```python
from build123d import *

# Parameters (mm, degrees)
SKETCH1_W                                    = 80
SKETCH1_H                                    = 225
BOSS_EXTRUDE1_DEPTH                          = 20
CUT_EXTRUDE1_REACH                           = 123.063
CUT_EXTRUDE2_DEPTH                           = 5
CBORE_FOR_M8_HEX_SOCKET_HEAD_CAP_SCR_2_COUNT = 2
CBORE_FOR_M8_HEX_SOCKET_HEAD_CAP_SCR_2_PITCH = 50
CBORE_FOR_M8_HEX_SOCKET_HEAD_CAP_SCR_3_COUNT = 2
CBORE_FOR_M8_HEX_SOCKET_HEAD_CAP_SCR_3_PITCH = 201.308221392
CBORE_FOR_M8_HEX_SOCKET_HEAD_CAP_SCR_4_COUNT = 2
CBORE_FOR_M8_HEX_SOCKET_HEAD_CAP_SCR_4_PITCH = 195
F_8_0MM_DOWEL_HOLE1_D                        = 8
SKETCH11_R                                   = 10
CUT_EXTRUDE3_DEPTH                           = 122.063000128
CUT_EXTRUDE4_REACH                           = 123.063
SKETCH13_R                                   = 6
CUT_EXTRUDE5_REACH                           = 123.063
SKETCH14_R                                   = 7


with BuildPart() as part:
    # Sketch1 → Boss-Extrude1 (new body)
    with BuildSketch(Plane(origin=(0, 0, 0), x_dir=(1, 0, 0), z_dir=(0, 1, 0))):
        Rectangle(SKETCH1_W, SKETCH1_H)
    extrude(amount=-BOSS_EXTRUDE1_DEPTH)

    # Sketch2 → Cut-Extrude1 (cut, up to next)
    with BuildSketch(Plane(origin=(0, 0, 0), x_dir=(1, 0, 0), z_dir=(0, 1, 0)), mode=Mode.PRIVATE) as cut_extrude1_sk1:
        with BuildLine():
            Line((24, 17.31), (24, 34.91))
            ThreePointArc((24, 34.91), (21.5, 37.41), (19, 34.91))
            Line((19, 34.91), (19, 17.31))
            ThreePointArc((19, 17.31), (21.5, 14.81), (24, 17.31))
        make_face()
    cut_extrude1_tool1 = extrude(cut_extrude1_sk1.sketch, amount=-CUT_EXTRUDE1_REACH, mode=Mode.PRIVATE) & part.part
    # Sketch2 → Cut-Extrude1 (cut, up to next)
    with BuildSketch(Plane(origin=(0, 0, 0), x_dir=(1, 0, 0), z_dir=(0, 1, 0)), mode=Mode.PRIVATE) as cut_extrude1_sk2:
        with BuildLine():
            Line((24, -36.69), (24, -12.59))
            ThreePointArc((24, -12.59), (21.5, -10.09), (19, -12.59))
            Line((19, -12.59), (19, -36.69))
            ThreePointArc((19, -36.69), (21.5, -39.19), (24, -36.69))
        make_face()
    cut_extrude1_tool2 = extrude(cut_extrude1_sk2.sketch, amount=-CUT_EXTRUDE1_REACH, mode=Mode.PRIVATE) & part.part
    # Sketch2 → Cut-Extrude1 (cut, up to next)
    with BuildSketch(Plane(origin=(0, 0, 0), x_dir=(1, 0, 0), z_dir=(0, 1, 0)), mode=Mode.PRIVATE) as cut_extrude1_sk3:
        with BuildLine():
            Line((-24, -16.59), (-24, -36.69))
            ThreePointArc((-24, -36.69), (-21.5, -39.19), (-19, -36.69))
            Line((-19, -36.69), (-19, -16.59))
            ThreePointArc((-19, -16.59), (-21.5, -14.09), (-24, -16.59))
        make_face()
    cut_extrude1_tool3 = extrude(cut_extrude1_sk3.sketch, amount=-CUT_EXTRUDE1_REACH, mode=Mode.PRIVATE) & part.part
    # Sketch2 → Cut-Extrude1 (cut, up to next)
    with BuildSketch(Plane(origin=(0, 0, 0), x_dir=(1, 0, 0), z_dir=(0, 1, 0)), mode=Mode.PRIVATE) as cut_extrude1_sk4:
        with BuildLine():
            Line((-24, 53.91), (-24, 36.31))
            ThreePointArc((-24, 36.31), (-21.5, 33.81), (-19, 36.31))
            Line((-19, 36.31), (-19, 53.91))
            ThreePointArc((-19, 53.91), (-21.5, 56.41), (-24, 53.91))
        make_face()
    cut_extrude1_tool4 = extrude(cut_extrude1_sk4.sketch, amount=-CUT_EXTRUDE1_REACH, mode=Mode.PRIVATE) & part.part
    add(cut_extrude1_tool1.solids().sort_by_distance((21.5, 0, -26.11))[0], mode=Mode.SUBTRACT)
    add(cut_extrude1_tool2.solids().sort_by_distance((21.5, 0, 24.64))[0], mode=Mode.SUBTRACT)
    add(cut_extrude1_tool3.solids().sort_by_distance((-21.5, 0, 26.64))[0], mode=Mode.SUBTRACT)
    add(cut_extrude1_tool4.solids().sort_by_distance((-21.5, 0, -45.11))[0], mode=Mode.SUBTRACT)

    # Sketch3 → Cut-Extrude2 (cut)
    with BuildSketch(Plane(origin=(0, 0, 0), x_dir=(1, 0, 0), z_dir=(0, 1, 0))):
        with BuildLine():
            Line((-17.5, 36.31), (-17.5, 53.91))
            ThreePointArc((-17.5, 53.91), (-21.5, 57.91), (-25.5, 53.91))
            Line((-25.5, 53.91), (-25.5, 36.31))
            ThreePointArc((-25.5, 36.31), (-21.5, 32.31), (-17.5, 36.31))
        make_face()
        with BuildLine():
            Line((25.5, 17.31), (25.5, 34.91))
            ThreePointArc((25.5, 34.91), (21.5, 38.91), (17.5, 34.91))
            Line((17.5, 34.91), (17.5, 17.31))
            ThreePointArc((17.5, 17.31), (21.5, 13.31), (25.5, 17.31))
        make_face()
        with BuildLine():
            Line((25.5, -36.69), (25.5, -12.59))
            ThreePointArc((25.5, -12.59), (21.5, -8.59), (17.5, -12.59))
            Line((17.5, -12.59), (17.5, -36.69))
            ThreePointArc((17.5, -36.69), (21.5, -40.69), (25.5, -36.69))
        make_face()
        with BuildLine():
            Line((-25.5, -16.59), (-25.5, -36.69))
            ThreePointArc((-25.5, -36.69), (-21.5, -40.69), (-17.5, -36.69))
            Line((-17.5, -36.69), (-17.5, -16.59))
            ThreePointArc((-17.5, -16.59), (-21.5, -12.59), (-25.5, -16.59))
        make_face()
    extrude(amount=-CUT_EXTRUDE2_DEPTH, mode=Mode.SUBTRACT)

    # Sketch6 → CBORE for M8 Hex Socket Head Cap Screw1 (revolve, cut)
    with BuildSketch(Plane(origin=(25, -20, -97.5), x_dir=(0, 0, -1), z_dir=(1, 0, 0))):
        Polygon((0, 0), (0, 20), (4.2, 20), (4.2, 8.6), (7.5, 8.6), (7.5, 0.025), (7.525, 0), align=None)
    cbore_for_m8_hex_socket_head_cap_screw1 = revolve(axis=Axis((25, -26.35, -97.5), (0, 1, 0)), mode=Mode.SUBTRACT)

    # CBORE for M8 Hex Socket Head Cap Scr 2: CBORE for M8 Hex Socket Head Cap Screw1 ×2
    with Locations(*[(-i * CBORE_FOR_M8_HEX_SOCKET_HEAD_CAP_SCR_2_PITCH, 0, 0) for i in range(1, CBORE_FOR_M8_HEX_SOCKET_HEAD_CAP_SCR_2_COUNT)]):
        add(cbore_for_m8_hex_socket_head_cap_screw1, mode=Mode.SUBTRACT)

    # CBORE for M8 Hex Socket Head Cap Scr 3: CBORE for M8 Hex Socket Head Cap Screw1 ×2
    with Locations(*[Vector(-0.24837535026770385, 0, 0.968663866044045) * (i * CBORE_FOR_M8_HEX_SOCKET_HEAD_CAP_SCR_3_PITCH) for i in range(1, CBORE_FOR_M8_HEX_SOCKET_HEAD_CAP_SCR_3_COUNT)]):
        add(cbore_for_m8_hex_socket_head_cap_screw1, mode=Mode.SUBTRACT)

    # CBORE for M8 Hex Socket Head Cap Scr 4: CBORE for M8 Hex Socket Head Cap Screw1 ×2
    with Locations(*[(0, 0, i * CBORE_FOR_M8_HEX_SOCKET_HEAD_CAP_SCR_4_PITCH) for i in range(1, CBORE_FOR_M8_HEX_SOCKET_HEAD_CAP_SCR_4_COUNT)]):
        add(cbore_for_m8_hex_socket_head_cap_screw1, mode=Mode.SUBTRACT)

    # Ø8.0mm Dowel Hole1 (through all)
    with Locations(Plane(origin=(0, -20, 0), x_dir=(-1, 0, 0), z_dir=(0, -1, 0))):
        with Locations((-25, 81.975), (25, -82)):
            Hole(F_8_0MM_DOWEL_HOLE1_D / 2)

    # Sketch11 → Cut-Extrude3 (cut, through all)
    with BuildSketch(Plane.XZ.offset(20)):
        with Locations(Location((-22, 55, 0), (0, 0, 270))):
            Circle(SKETCH11_R)
        with Locations(Location((22, 55, 0), (0, 0, 270))):
            Circle(SKETCH11_R)
        with Locations(Location((-22, -72, 0), (0, 0, 270))):
            Circle(SKETCH11_R)
        with Locations(Location((22, -60, 0), (0, 0, 270))):
            Circle(SKETCH11_R)
        with Locations(Location((0, -35, 0), (0, 0, 270))):
            Circle(SKETCH11_R)
        with Locations(Location((0, 25, 0), (0, 0, 270))):
            Circle(SKETCH11_R)
    extrude(amount=-CUT_EXTRUDE3_DEPTH, mode=Mode.SUBTRACT)

    # Sketch13 → Cut-Extrude4 (cut, up to next)
    with BuildSketch(Plane(origin=(0, 0, 0), x_dir=(1, 0, 0), z_dir=(0, 1, 0)), mode=Mode.PRIVATE) as cut_extrude4_sk1:
        with Locations(Location((0, 100, 0), (0, 0, 270))):
            Circle(SKETCH13_R)
    cut_extrude4_tool1 = extrude(cut_extrude4_sk1.sketch, amount=-CUT_EXTRUDE4_REACH, mode=Mode.PRIVATE) & part.part
    # Sketch13 → Cut-Extrude4 (cut, up to next)
    with BuildSketch(Plane(origin=(0, 0, 0), x_dir=(1, 0, 0), z_dir=(0, 1, 0)), mode=Mode.PRIVATE) as cut_extrude4_sk2:
        with Locations(Location((0, -100, 0), (0, 0, 270))):
            Circle(SKETCH13_R)
    cut_extrude4_tool2 = extrude(cut_extrude4_sk2.sketch, amount=-CUT_EXTRUDE4_REACH, mode=Mode.PRIVATE) & part.part
    # Sketch13 → Cut-Extrude4 (cut, up to next)
    with BuildSketch(Plane(origin=(0, 0, 0), x_dir=(1, 0, 0), z_dir=(0, 1, 0)), mode=Mode.PRIVATE) as cut_extrude4_sk3:
        with Locations(Location((-30, 4, 0), (0, 0, 270))):
            Circle(SKETCH13_R)
    cut_extrude4_tool3 = extrude(cut_extrude4_sk3.sketch, amount=-CUT_EXTRUDE4_REACH, mode=Mode.PRIVATE) & part.part
    # Sketch13 → Cut-Extrude4 (cut, up to next)
    with BuildSketch(Plane(origin=(0, 0, 0), x_dir=(1, 0, 0), z_dir=(0, 1, 0)), mode=Mode.PRIVATE) as cut_extrude4_sk4:
        with Locations(Location((30, 4, 0), (0, 0, 270))):
            Circle(SKETCH13_R)
    cut_extrude4_tool4 = extrude(cut_extrude4_sk4.sketch, amount=-CUT_EXTRUDE4_REACH, mode=Mode.PRIVATE) & part.part
    add(cut_extrude4_tool1.solids().sort_by_distance((0, 0, -100))[0], mode=Mode.SUBTRACT)
    add(cut_extrude4_tool2.solids().sort_by_distance((0, 0, 100))[0], mode=Mode.SUBTRACT)
    add(cut_extrude4_tool3.solids().sort_by_distance((-30, 0, -4))[0], mode=Mode.SUBTRACT)
    add(cut_extrude4_tool4.solids().sort_by_distance((30, 0, -4))[0], mode=Mode.SUBTRACT)

    # Sketch14 → Cut-Extrude5 (cut, up to next)
    with BuildSketch(Plane(origin=(0, 0, 0), x_dir=(1, 0, 0), z_dir=(0, 1, 0)), mode=Mode.PRIVATE) as cut_extrude5_sk1:
        with Locations(Location((0, 9.86, 0), (0, 0, 270))):
            Circle(SKETCH14_R)
    cut_extrude5_tool1 = extrude(cut_extrude5_sk1.sketch, amount=-CUT_EXTRUDE5_REACH, mode=Mode.PRIVATE) & part.part
    add(cut_extrude5_tool1.solids().sort_by_distance((0, 0, -9.86))[0], mode=Mode.SUBTRACT)


solid = part.part
```
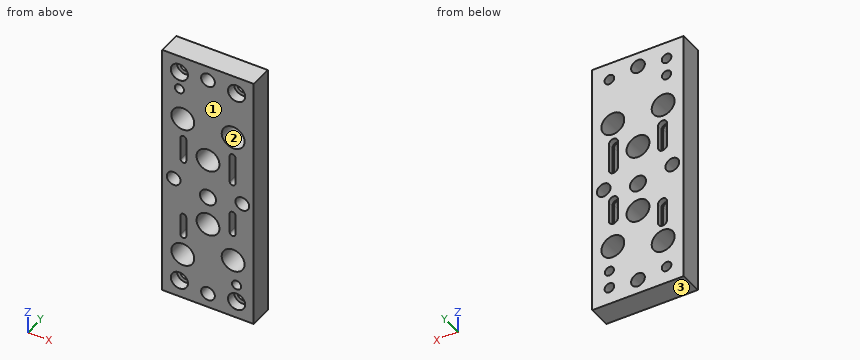
Could you check a few things on this model? Use its own coordinates, in mm. Face numbers are marked on the shaded views. Round coordinates to 2 decimals unless told otherwise and drop trailing zeros. Write each loop counter-clockwise with the first axis right and the second up, starting at its lowest first coordinate (ties: lowest second). Pieces come first, ordered by that corner, then holes.
(1) Suppose I cut it at A-A on z = -60. Write out the boundary of the cut face in (x, y), and give its area (3 significant figures).
Findings below:
outline: (-40, -20) - (12, -20) - (12, 0) - (-40, 0) - close; (32, -20) - (40, -20) - (40, 0) - (32, 0) - close
area: 1,200 mm2
(2) Suppose I cut it at C-C on x = -3. Write out the boundary of the cut face in (y, z), and give its area (3 significant figures).
Findings below:
outline: (-20, -112.5) - (0, -112.5) - (0, -105.2) - (-20, -105.2) - close; (-20, -94.8) - (0, -94.8) - (0, -44.54) - (-20, -44.54) - close; (-20, -25.46) - (0, -25.46) - (0, -16.18) - (-20, -16.18) - close; (-20, -3.54) - (0, -3.54) - (0, 15.46) - (-20, 15.46) - close; (-20, 34.54) - (0, 34.54) - (0, 94.8) - (-20, 94.8) - close; (-20, 105.2) - (0, 105.2) - (0, 112.5) - (-20, 112.5) - close
area: 3,070 mm2
(3) For pin 1 (9.5 mm diameter, centred on x = -25, z = 97.5, fed in from -Y); pin 2 (6.5 mm diameter, centred on x = -19.5, z = 29.5, fed in from +Y), each with a flat end and sliding along its axis, tell me the tip position at first contact or that it passes through.
Findings below:
pin 1: stops at y = -11.4
pin 2: stops at y = 0
(4) If I drill on probe 1 along X at (y, z) = (-17.75, -27); probe 2 along X at (y, z) = (-14.5, 55); probe 3 along X at (y, z) = (-11.5, 12.5), over which ranges is the centre line in solid material (lowest first)?
Findings below:
probe 1: x = -40 to -6, 6 to 19, 24 to 40
probe 2: x = -40 to -32, -12 to 12, 32 to 40
probe 3: x = -40 to 19, 24 to 40
(5) Thinking about a two-plate mould opening in Z: for the marked faces 1, 2 and 3, which applies, +Z half, -Z half, draft (parallel to the pull), parting line (faces both ways), or undercut?
Findings below:
face 1: draft
face 2: undercut
face 3: -Z half
(6) Suppose I cut it at B-B on z = 25. Write out the boundary of the cut face in (x, y), and give its area (3 significant figures).
Findings below:
outline: (-40, -20) - (-24, -20) - (-24, -5) - (-25.5, -5) - (-25.5, 0) - (-40, 0) - close; (-19, -20) - (-10, -20) - (-10, 0) - (-17.5, 0) - (-17.5, -5) - (-19, -5) - close; (10, -20) - (19, -20) - (19, -5) - (17.5, -5) - (17.5, 0) - (10, 0) - close; (24, -20) - (40, -20) - (40, 0) - (25.5, 0) - (25.5, -5) - (24, -5) - close
area: 970 mm2
(7) Suppose I cut it at D-D on y = -7.75. State how many separate pieces and enclosed holes the cut face has, and give its area (3 significant figures).
Findings below:
separate pieces: 1
enclosed holes: 21
area: 14,700 mm2
